from build123d import *

# Parameters (mm, degrees)
F1_DEPTH = 10


# Not quite as in the source:
# - a feature names something its author has since deleted; it is built from what else it names


with BuildPart() as f1:
    # F0 (on Front) → F1 (new body)
    with BuildSketch(Plane.XZ):
        with BuildLine():
            Line((-152.9289321881, 147.0710678119), (-300, 0))
            Line((-300, 0), (-381.3172798365, -81.3172798365))
            ThreePointArc((-381.3172798365, -81.3172798365), (-384.2462120246, -88.3883476483), (-381.3172798365, -95.4594154602))
            Line((-381.3172798365, -95.4594154602), (-155.0431098568, -321.7335854399))
            Line((-155.0431098568, -321.7335854399), (-7.0710678119, -469.7056274848))
            ThreePointArc((-7.0710678119, -469.7056274848), (0, -472.6345596729), (7.0710678119, -469.7056274848))
            Line((7.0710678119, -469.7056274848), (155.0431098568, -321.7335854399))
            Line((155.0431098568, -321.7335854399), (381.3172798365, -95.4594154602))
            ThreePointArc((381.3172798365, -95.4594154602), (384.2462120246, -88.3883476483), (381.3172798365, -81.3172798365))
            Line((381.3172798365, -81.3172798365), (300, 0))
            Line((300, 0), (152.9289321881, 147.0710678119))
            ThreePointArc((152.9289321881, 147.0710678119), (149.6846986999, 149.2387953251), (145.8578643763, 150))
            Line((145.8578643763, 150), (-145.8578643763, 150))
            ThreePointArc((-145.8578643763, 150), (-149.6846986999, 149.2387953251), (-152.9289321881, 147.0710678119))
        make_face()
    extrude(amount=F1_DEPTH)


solid = f1.part
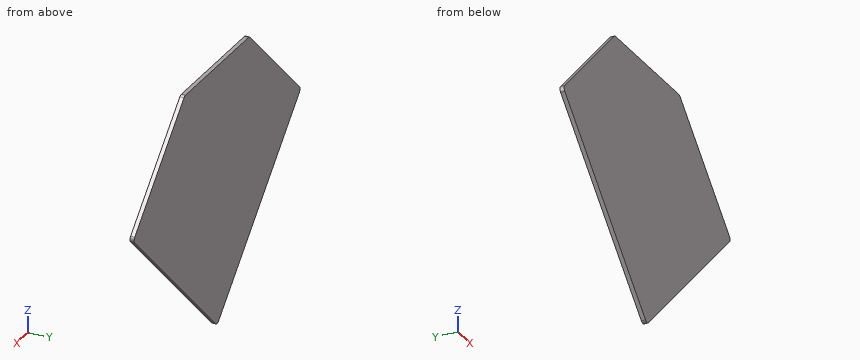
Read the model definition and answer for the solid it produces. Units are mm, in the model's axes. Give positions to 0.01 mm unless a question says otherwise; leave off trailing zeros. Write each loop counter-clockwise with the first axis right and the second up, starting at its lowest first coordinate (ties: lowest second). Pieces come first, ordered by that corner, then holes. Notation, with made-up numbers: (-25.5, 78.25) - (-0.5, 78.25) arc R4 cw to (-0.5, 85.25) - close; hole circle Ø3 at (37.25, -21.75). An arc over 180 degrees is marked (long way). Use CSV: the item, a comma, the result in double quotes. Start each with the question number.
Item 1: The part is cut by section B-B, the plane z = 41.5. Give the vertices of the cut face in (x, y), and give its area (3 significant figures).
Item 2: The part is cut by section C-C, the plane x = 178. Give the vertices of the cut face in (y, z).
Item 3: The part is cut by section A-A, the plane y = -2.75. Give the vertices of the cut face in (x, z).
Item 4: Flat-ended cylindrical pins translate along their axes: P1, Ø12, axis at x = -304, z = -4.5, coming from the +Y side; P2, Ø1.5, axis at y = -2.5, z = -202.5, coming from the -X side; P3, Ø1.5, axis at x = -252, y = -6, coming from the -Z side; P4, Ø2, axis at y = -1.5, z = -285, coming from the +X side. Find the tip coordinate at first contact, or state that the pin passes through.
Item 5: Consider line 1 (Z direction, x = -199, y = -5); line 2 (X direction, y = -6.25, z = -356); line 3 (Z direction, x = 299, y = -4.25). Determine where each line is inside the solid, lowest interval first.
Taken from the geometry:
1,outline,"(-258.5, -10) - (258.5, -10) - (258.5, 0) - (-258.5, 0) - close"
1,area,"5,170 mm2"
2,outline,"(-10, -298.78) - (0, -298.78) - (0, 122) - (-10, 122) - close"
3,outline,"(-381.32, -95.46) - (-7.07, -469.71) arc R10 ccw to (7.07, -469.71) - (381.32, -95.46) arc R10 ccw to (381.32, -81.32) - (152.93, 147.07) arc R10 ccw to (145.86, 150) - (-145.86, 150) arc R10 ccw to (-152.93, 147.07) - (-381.32, -81.32) arc R10 ccw to start"
4,P1,"y = 0"
4,P2,"x = -275.03"
4,P3,"z = -225.53"
4,P4,"x = 192.78"
5,line 1,"-277.78 to 101"
5,line 2,"-120.78 to 120.78"
5,line 3,"-177.78 to 1"
